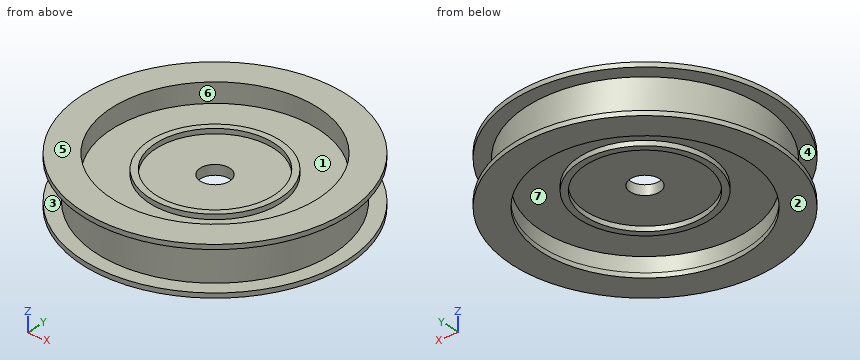
```python
from build123d import *

# Parameters (mm, degrees)
SKETCH1_R           = 19.05
BOSS_EXTRUDE1_DEPTH = 0.79375
SKETCH3_R           = 19.05
SKETCH3_R_2         = 16.637
BOSS_EXTRUDE2_DEPTH = 3.175
SKETCH4_R           = 10.541
SKETCH4_R_2         = 9.525
BOSS_EXTRUDE3_DEPTH = 1.5875
SKETCH6_R           = 2.38125
CUT_EXTRUDE4_DEPTH  = 28.231525417
SKETCH7_R           = 21.336
SKETCH7_R_2         = 16.637
BOSS_EXTRUDE5_DEPTH = 0.762


with BuildPart() as part:
    # Sketch1 → Boss-Extrude1 (new, symmetric)
    with BuildSketch(Plane.XY):
        Circle(SKETCH1_R)
    extrude(amount=BOSS_EXTRUDE1_DEPTH, both=True)

    # Sketch3 → Boss-Extrude2 (add, symmetric)
    with BuildSketch(Plane.XY):
        Circle(SKETCH3_R)
        Circle(SKETCH3_R_2, mode=Mode.SUBTRACT)
    extrude(amount=BOSS_EXTRUDE2_DEPTH, both=True)

    # Sketch4 → Boss-Extrude3 (add, symmetric)
    with BuildSketch(Plane.XY):
        Circle(SKETCH4_R)
        Circle(SKETCH4_R_2, mode=Mode.SUBTRACT)
    extrude(amount=BOSS_EXTRUDE3_DEPTH, both=True)

    # Sketch6 → Cut-Extrude4 (cut, through all)
    with BuildSketch(Plane.XY.offset(0.79375)):
        Circle(SKETCH6_R)
    extrude(amount=-CUT_EXTRUDE4_DEPTH, mode=Mode.SUBTRACT)

    # Sketch7 → Boss-Extrude5 (add)
    with BuildSketch(Plane.XY.offset(3.175)):
        with Locations(Location((0, 0, 0), (0, 0, 180))):
            Circle(SKETCH7_R)
        Circle(SKETCH7_R_2, mode=Mode.SUBTRACT)
    boss_extrude5 = extrude(amount=BOSS_EXTRUDE5_DEPTH)

    # Mirror3: Boss-Extrude5 across plane
    add(boss_extrude5.mirror(Plane.XY))


solid = part.part
```
Can you work these out from the model? Positions are in its coordinate system, mm. Face numbers are marked on the shaded views. A direction names the side the tool comes from. Round coordinates to 2 decimals unless told otherwise and drop trailing zeros. Order: outer loops, then holes, each group sorted by start corner. A loop starts at its lowest first (then second) coordinate and runs counter-clockwise, first axis right, second up.
(1) If we section it at D-D (z = -0.25): Please give me the cut outline in (x, y).
Results are:
outline: circle Ø38.1 at (0, 0); hole circle Ø4.76 at (0, 0)
(2) We'd pull the mould along Z, two halves only. Please class the marked faces 1, 2 and 3: +Z half, -Z half, draft (parallel to the pull), parting line (faces both ways), or undercut.
Results are:
face 1: +Z half
face 2: -Z half
face 3: undercut
(3) On a 3-axis mill with a long thin cutter (end or side, diameter ignored), from which of +Z, -Z, +X, -X, +Y, -Y can I reach the whole of each face in a straight line? I mean the marked faces 4, 5, 6 and 7. Say none if no direction works.
Results are:
face 4: none
face 5: +Z, +X, -X, +Y, -Y
face 6: +Z
face 7: -Z
(4) If we section it at A-A (z = 2.5): Please give me the cut outline in (x, y), plus the area to 3 significant figures.
Results are:
outline: circle Ø38.1 at (0, 0); hole circle Ø33.27 at (0, 0)
area: 271 mm2
(5) If I drill on L1, parallel to Y at x = 0, z = 1 (3 decimals); L2, parallel to Z at x = -7, y = -19 (3 decimals); L3, parallel to Y at x = 0, z = -3.6, over which ranges is the centre line in solid material (lowest first)?
Results are:
L1: y = -19.05 to -16.637, -10.541 to -9.525, 9.525 to 10.541, 16.637 to 19.05
L2: z = -3.937 to -3.175, 3.175 to 3.937
L3: y = -21.34 to -16.64, 16.64 to 21.34
(6) If we section it at C-C (x = -17.5): Please give me the cut outline in (y, z) (3 decimals), plus the area to 3 significant figures.
Results are:
outline: (-12.206, -3.937) - (12.206, -3.937) - (12.206, -3.175) - (7.527, -3.175) - (7.527, 3.175) - (12.206, 3.175) - (12.206, 3.937) - (-12.206, 3.937) - (-12.206, 3.175) - (-7.527, 3.175) - (-7.527, -3.175) - (-12.206, -3.175) - close
area: 133 mm2
(7) I'm going to push flat-ended pins straight in: pin 1 (15 mm diameter, centred on x = 0, y = 0, fed in from -Z); pin 2 (23 mm diameter, centred on x = -1.5, y = 1.5, fed in from +Z); pin 3 (1 mm diameter, centred on y = -9.5, z = -2.5, fed in from -X); pin 4 (4 mm diameter, centred on x = 0, y = 0, fed in from -Z). Where does each tip first touch, or does it pass through?
Results are:
pin 1: stops at z = -0.79
pin 2: stops at z = 1.59
pin 3: stops at x = -16.79
pin 4: passes through
(8) If we section it at B-B (y = -16): Please give me the cut outline in (x, z) (3 decimals).
Results are:
outline: (-14.115, -3.937) - (-4.56, -3.937) - (-4.56, -0.794) - (4.56, -0.794) - (4.56, -3.937) - (14.115, -3.937) - (14.115, -3.175) - (10.339, -3.175) - (10.339, 3.175) - (14.115, 3.175) - (14.115, 3.937) - (4.56, 3.937) - (4.56, 0.794) - (-4.56, 0.794) - (-4.56, 3.937) - (-14.115, 3.937) - (-14.115, 3.175) - (-10.339, 3.175) - (-10.339, -3.175) - (-14.115, -3.175) - close
